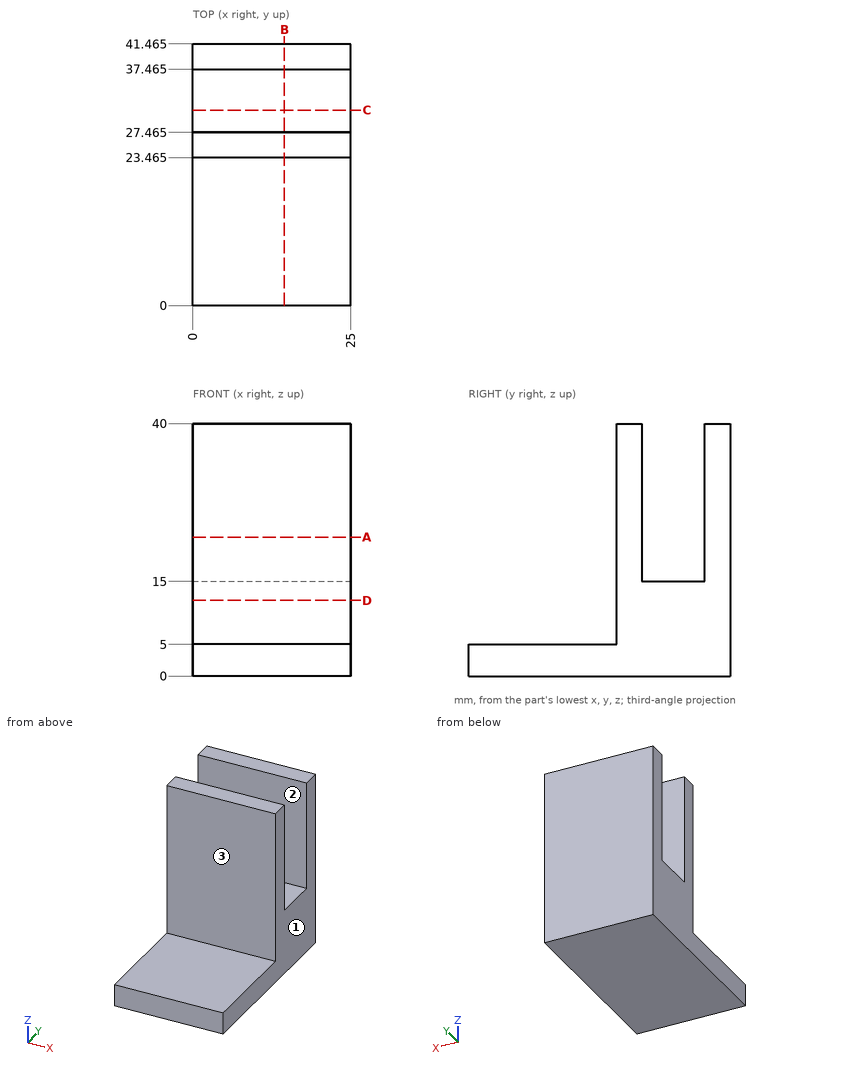
Geometry: see drawing. Coordinates: mm, zero at the bounding-box minimum. A direction names the side the tool comes from. Coordinates: 2 decimals unless noted, no trailing zeros. Loops run counter-clockwise (first coordinate to the right, second up) from the corner with the lowest first, then second, coordinate; pieces in that order, holes last. Notation, with made-up numbers: (18.25, 28.5) -> (47.25, 28.5) arc R14 ccw to (47.25, 50.5) -> close; hole circle Ø4 at (86, -34.5). An arc over 180 degrees is marked (long way). Write item = value, one per line. Start each with the question number.
Item 1: Cut plane A-A, the plane z = 22. Return loops of the section in (x, y) (1 decimal).
Item 2: First-contact query: P1, Ø4, axis at x = 10, z = 12.5, coming from the -Y side (1 decimal); P2, Ø5, axis at x = 9, y = 31, coming from the +Z side. Flat tips, straight axial feed; report the tip coordinate or a pass-through.
Item 3: Reachability of the marked faces 1, 2 and 3 from +Z, -Z, +X, -X, +Y, -Y: full face, straight path, thin tool, end or side. Return the list, or none.
Item 4: Cut plane B-B, the plane x = 14.5. Return loops of the section in (y, z) (1 decimal).
Item 5: Cut plane C-C, the plane y = 31. Return loops of the section in (x, z), plus the area to 3 significant figures.
Item 6: Material intervals for line 1 (Y direction, x = 13, z = 26) (1 decimal); line 2 (Y direction, x = 18, z = 6) (1 decimal); line 3 (Z direction, x = 19.25, y = 28), sorted ascending.
Item 7: Cut plane D-D, the plane z = 12. Return loops of the section in (x, y) (1 decimal).
Ans:
q1.outline = (0, 23.5) -> (25, 23.5) -> (25, 27.5) -> (0, 27.5) -> close; (0, 37.5) -> (25, 37.5) -> (25, 41.5) -> (0, 41.5) -> close
q2.P1 = 23.5
q2.P2 = 15
q3.face_1 = +Z, -Z, +X, +Y, -Y
q3.face_2 = +Z, +X, -X
q3.face_3 = +Z, +X, -X, -Y
q4.outline = (0, 0) -> (41.5, 0) -> (41.5, 40) -> (37.5, 40) -> (37.5, 15) -> (27.5, 15) -> (27.5, 40) -> (23.5, 40) -> (23.5, 5) -> (0, 5) -> close
q5.outline = (0, 0) -> (25, 0) -> (25, 15) -> (0, 15) -> close
q5.area = 375 mm²
q6.line_1 = 23.5 to 27.5, 37.5 to 41.5
q6.line_2 = 23.5 to 41.5
q6.line_3 = 0 to 15
q7.outline = (0, 23.5) -> (25, 23.5) -> (25, 41.5) -> (0, 41.5) -> close
